```python
from build123d import *

# Parameters (mm, degrees)
SKETCH_1_W      = 13.300240072
SKETCH_1_H      = 33.5
EXTRUDE_1_DEPTH = 3


with BuildPart() as part:
    # ｽｹｯﾁ1 → ﾎﾞｽ - 押し出し1 (new body)
    with BuildSketch(Plane.XY):
        with BuildLine():
            Line((-1.634343126, 16.855350031), (-7.977588702, 26.788033743))
            ThreePointArc((-7.977588702, 26.788033743), (-9.854266456, 28.542819322), (-12.343280841, 29.18))
            Line((-12.343280841, 29.18), (-29.549149223, 29.18))
            ThreePointArc((-29.549149223, 29.18), (-32.106762662, 28.50455475), (-33.997376931, 26.654368145))
            Line((-33.997376931, 26.654368145), (-42.448262973, 12.492253701))
            ThreePointArc((-42.448262973, 12.492253701), (-42.993742281, 11.214580959), (-43.180035265, 9.837885555))
            Line((-43.180035265, 9.837885555), (-43.180035265, -15.34473303))
            ThreePointArc((-43.180035265, -15.34473303), (-42.993742281, -16.721428434), (-42.448262973, -17.999101176))
            Line((-42.448262973, -17.999101176), (-33.997376931, -32.16121562))
            ThreePointArc((-33.997376931, -32.16121562), (-32.106762662, -34.011402225), (-29.549149223, -34.686847475))
            Line((-29.549149223, -34.686847475), (-12.343280841, -34.686847475))
            ThreePointArc((-12.343280841, -34.686847475), (-9.854266456, -34.049666797), (-7.977588702, -32.294881217))
            Line((-7.977588702, -32.294881217), (-1.634343126, -22.362197506))
            ThreePointArc((-1.634343126, -22.362197506), (-1.027777967, -21.026423162), (-0.820035265, -19.574163763))
            Line((-0.820035265, -19.574163763), (-0.820035265, 14.067316288))
            ThreePointArc((-0.820035265, 14.067316288), (-1.027777967, 15.519575687), (-1.634343126, 16.855350031))
        make_face()
        with Locations((-16.499940321, 4.15)):
            Rectangle(SKETCH_1_W, SKETCH_1_H, mode=Mode.SUBTRACT)
    extrude(amount=EXTRUDE_1_DEPTH)


solid = part.part
```
Part model, mm, in its own coordinate system. A direction names the side the tool comes from. Coordinates: 2 decimals unless noted, no trailing zeros. Write each loop counter-clockwise with the first axis right and the second up, starting at its lowest first coordinate (ties: lowest second). Pieces come first, ordered by that corner, then holes.
Item 1: Mould opens along Y. For faces 3 (the face through (-17, 20.9, 1)), 4 (the face through (-4.85, -27.4, 1.48)), 5 (the face through (-27, -2, 0)) say: released by +Y, released by -Y, zero draft, split by the parting line, or undercut.
Item 2: Slice it at D-D (x = -7). Write the cut outline in (y, z), and give its area (3 significant figures).
Item 3: Slice it at A-A (y = -1). Write the cut outline in (x, z), and give its area (3 significant figures).
Item 4: Probe line 1 (Y direction, x = -12.5, z = 2.1); line 2 (X direction, y = 7.5, z = 2.85); line 3 (Y direction, x = -34, z = 2.1). List the from-to ranges inside material, lowest first.
Item 5: Slice it at C-C (x = -21.5). Write the cut outline in (y, z), and give its area (3 significant figures).
Item 6: Slice it at B-B (z = 0.5). Write the cut outline in (x, y), and give its area (3 significant figures).
Item 7: Which spindle directions (+Z, -Z, +X, -X, +Y, -Y) get a long thin tool onto all of the face, cutting with end or side? Do faces 1 (the face through (-9.822, 28.525, 1.479)), 2 (the face through (-17, -12.6, 1)). Say none if no direction does.
Results found:
1. face 3: undercut
1. face 4: released by -Y
1. face 5: zero draft
2. outline: (-30.76, 0) - (25.26, 0) - (25.26, 3) - (-30.76, 3) - close
2. area: 168 mm2
3. outline: (-43.18, 0) - (-23.15, 0) - (-23.15, 3) - (-43.18, 3) - close; (-9.85, 0) - (-0.82, 0) - (-0.82, 3) - (-9.85, 3) - close
3. area: 87.2 mm2
4. line 1: y = -34.69 to -12.6, 20.9 to 29.18
4. line 2: x = -43.18 to -23.15, -9.85 to -0.82
4. line 3: y = -32.16 to 26.65
5. outline: (-34.69, 0) - (-12.6, 0) - (-12.6, 3) - (-34.69, 3) - close; (20.9, 0) - (29.18, 0) - (29.18, 3) - (20.9, 3) - close
5. area: 91.1 mm2
6. outline: (-43.18, -15.34) arc R5.18 ccw to (-42.45, -18) - (-34, -32.16) arc R5.18 ccw to (-29.55, -34.69) - (-12.34, -34.69) arc R5.18 ccw to (-7.98, -32.29) - (-1.63, -22.36) arc R5.18 ccw to (-0.82, -19.57) - (-0.82, 14.07) arc R5.18 ccw to (-1.63, 16.86) - (-7.98, 26.79) arc R5.18 ccw to (-12.34, 29.18) - (-29.55, 29.18) arc R5.18 ccw to (-34, 26.65) - (-42.45, 12.49) arc R5.18 ccw to (-43.18, 9.84) - close; hole (-23.15, -12.6) - (-9.85, -12.6) - (-9.85, 20.9) - (-23.15, 20.9) - close
6. area: 1,940 mm2
7. face 1: +Z, -Z, +X, +Y
7. face 2: +Z, -Z
